Source: CAD feature listing. Evaluate the final solid. Frame: model axes, mm. A direction names the side the tool comes from. Round coordinates to 2 decimals unless told otherwise and drop trailing zeros. Write each loop counter-clockwise with the first axis right and the second up, starting at its lowest first coordinate (ties: lowest second). Pieces come first, ordered by that corner, then holes. Notation, with made-up numbers: (87.5, 49) -> (114.5, 49) arc R10 cw to (114.5, 64) -> close; hole circle Ø11 at (41.25, -0.75). An arc over 180 degrees is marked (long way). Put each result on its own line as item: value.
```python
from build123d import *

# Parameters (mm, degrees)
ESQUISSE1_W               = 60.5
ESQUISSE1_H               = 64
BOSS_EXTRU_1_DEPTH        = 30
ESQUISSE2_R               = 4.5
ENL_V_MAT_EXTRU_1_DEPTH   = 32
ENL_V_MAT_EXTRU_2_REACH   = 55.283
ESQUISSE4_W               = 52.1
ESQUISSE4_H               = 83.557669167
ESQUISSE5_R               = 10.5
ENL_V_MAT_EXTRU_3_DEPTH   = 1.7
ESQUISSE6_R               = 10
ENL_V_MAT_EXTRU_4_DEPTH   = 4.2
ESQUISSE7_W               = 47
ESQUISSE7_H               = 57
BOSS_EXTRU_2_DEPTH        = 30
ENL_V_MAT_EXTRU_5_DEPTH   = 30
ENL_V_MAT_EXTRU_6_DEPTH   = 8.25
ESQUISSE11_W              = 5
ESQUISSE11_H              = 40.5
BOSS_EXTRU_3_DEPTH        = 5
ESQUISSE12_R              = 0.5
ENL_V_MAT_EXTRU_7_DEPTH   = 15
TROU_TARAUD_M2X0_42_D     = 1.6
TROU_TARAUD_M2X0_42_DEPTH = 17
TROU_TARAUD_M2X0_42_TIP   = 0.480688495
ENL_V_MAT_EXTRU_8_REACH   = 113.72
TROU_TARAUD_M3X0_54_D     = 2.5
TROU_TARAUD_M3X0_54_DEPTH = 17.5
TROU_TARAUD_M3X0_54_TIP   = 0.751075774
ENL_V_MAT_EXTRU_9_REACH   = 100.671
ESQUISSE26_W              = 5
ESQUISSE26_H              = 64.513244551
BOSS_EXTRU_5_START        = 0.8
BOSS_EXTRU_5_DEPTH        = 0.8
BOSS_EXTRU_6_DEPTH        = 0.5
ESQUISSE30_R              = 10
ENL_V_MAT_EXTRU_10_DEPTH  = 20.5
ENL_V_START               = -20.5
ESQUISSE32_R              = 10.5
ENL_V_MAT_EXTRU_13_DEPTH  = 20.5


with BuildPart() as part:
    # Esquisse1 → Boss.-Extru.1 (new body)
    with BuildSketch(Plane.XY):
        Rectangle(ESQUISSE1_W, ESQUISSE1_H)
    extrude(amount=BOSS_EXTRU_1_DEPTH)

    # Esquisse2 → Enlèv. mat.-Extru.1 (cut)
    with BuildSketch(Plane(origin=(30.25, 0, 0), x_dir=(0, 0, -1), z_dir=(1, 0, 0))):
        with Locations(Location((-15, -17, 0), (0, 0, 90))):
            Circle(ESQUISSE2_R)
    extrude(amount=-ENL_V_MAT_EXTRU_1_DEPTH, mode=Mode.SUBTRACT)

    # Enlèv. mat.-Extru.2: up to this face of the body (flat: up to its plane)
    enl_v_mat_extru_2_end = Plane(part.part.faces().sort_by_distance((0, 0, 0))[0])
    # Esquisse4 → Enlèv. mat.-Extru.2 (cut, up to the picked face)
    with BuildSketch(Plane.XY.offset(30), mode=Mode.PRIVATE) as enl_v_mat_extru_2_sk1:
        with Locations((0, -14.778834584)):
            Rectangle(ESQUISSE4_W, ESQUISSE4_H)
    enl_v_mat_extru_2_tool1 = split(extrude(enl_v_mat_extru_2_sk1.sketch, amount=-ENL_V_MAT_EXTRU_2_REACH, mode=Mode.PRIVATE), bisect_by=enl_v_mat_extru_2_end, keep=Keep.BOTH, mode=Mode.PRIVATE)
    add(enl_v_mat_extru_2_tool1.solids().sort_by(Axis((0, -14.778835, 30), (0, 0, -1)))[0], mode=Mode.SUBTRACT)

    # Esquisse5 → Enlèv. mat.-Extru.3 (cut)
    with BuildSketch(Plane(origin=(30.25, 0, 0), x_dir=(0, 0, -1), z_dir=(1, 0, 0))):
        with Locations(Location((-15, -17, 0), (0, 0, 90))):
            Circle(ESQUISSE5_R)
    extrude(amount=-ENL_V_MAT_EXTRU_3_DEPTH, mode=Mode.SUBTRACT)

    # Esquisse6 → Enlèv. mat.-Extru.4 (cut)
    with BuildSketch(Plane(origin=(-26.05, 0, 0), x_dir=(0, 0, -1), z_dir=(1, 0, 0))):
        with Locations((-15, -17)):
            Circle(ESQUISSE6_R)
    extrude(amount=-ENL_V_MAT_EXTRU_4_DEPTH, mode=Mode.SUBTRACT)

    # Esquisse7 → Boss.-Extru.2 (add)
    with BuildSketch(Plane.XY.offset(30)):
        with Locations((-6.75, 60.5)):
            Rectangle(ESQUISSE7_W, ESQUISSE7_H)
    extrude(amount=-BOSS_EXTRU_2_DEPTH)

    # Esquisse8 → Enlèv. mat.-Extru.5 (cut)
    with BuildSketch(Plane.XY.offset(30)):
        Polygon((-15.25, 80.75), (11.75, 80.75), (11.75, 98.556441221), (21.75, 98.556441221), (21.75, 32), (11.75, 32), (11.75, 40.25), (-15.25, 40.25), align=None)
    extrude(amount=-ENL_V_MAT_EXTRU_5_DEPTH, mode=Mode.SUBTRACT)

    # Esquisse10 → Enlèv. mat.-Extru.6 (cut)
    with BuildSketch(Plane.XZ.offset(-80.75)):
        Polygon((-5.25, 11), (-5.25, 12), (34.75, 12), (34.75, 18), (-5.25, 18), (-5.25, 19), (-15.25, 19), (-15.25, 11), align=None)
    extrude(amount=-ENL_V_MAT_EXTRU_6_DEPTH, mode=Mode.SUBTRACT)

    # Esquisse11 → Boss.-Extru.3 (add)
    with BuildSketch(Plane(origin=(-15.25, 0, 0), x_dir=(0, 0, -1), z_dir=(1, 0, 0))):
        with Locations((-27.5, 60.5)):
            Rectangle(ESQUISSE11_W, ESQUISSE11_H)
        with Locations((-2.5, 60.5)):
            Rectangle(ESQUISSE11_W, ESQUISSE11_H)
    extrude(amount=BOSS_EXTRU_3_DEPTH)

    # Esquisse12 → Enlèv. mat.-Extru.7 (cut)
    with BuildSketch(Plane(origin=(11.75, 0, 0), x_dir=(0, 0, -1), z_dir=(1, 0, 0))):
        with Locations((-19.925, 85.21)):
            Circle(ESQUISSE12_R)
        with Locations(Location((-10.075, 85.21, 0), (0, 0, 180))):
            Circle(ESQUISSE12_R)
        with Locations((-10.075, 35.79)):
            Circle(ESQUISSE12_R)
        with Locations(Location((-19.925, 35.79, 0), (0, 0, 180))):
            Circle(ESQUISSE12_R)
    extrude(amount=-ENL_V_MAT_EXTRU_7_DEPTH, mode=Mode.SUBTRACT)

    # Trou taraudé M2x0.42
    with Locations(Plane(origin=(11.75, 85.21, 19.925), x_dir=(0, 0, 1), z_dir=(1, 0, 0))):
        with Locations((0, 0), (-9.85, 0), (-9.85, 49.42), (0, 49.42)):
            Hole(TROU_TARAUD_M2X0_42_D / 2, depth=TROU_TARAUD_M2X0_42_DEPTH)
            with Locations((0, 0, -(TROU_TARAUD_M2X0_42_DEPTH + TROU_TARAUD_M2X0_42_TIP / 2))):  # 118° drill point
                Cone(0, TROU_TARAUD_M2X0_42_D / 2, TROU_TARAUD_M2X0_42_TIP, mode=Mode.SUBTRACT)

    # Enlèv. mat.-Extru.8: up to this face of the body (flat: up to its plane)
    enl_v_mat_extru_8_end = Plane(part.part.faces().sort_by_distance((30.25, 3.741727612, 15))[0])
    # Esquisse15 → Enlèv. mat.-Extru.8 (cut, up to the picked face)
    with BuildSketch(Plane.ZY.offset(30.25), mode=Mode.PRIVATE) as enl_v_mat_extru_8_sk1:
        with BuildLine():
            Line((40, -17), (30, -17))
            ThreePointArc((30, -17), (15, -32), (0, -17))
            Line((0, -17), (-10, -17))
            ThreePointArc((-10, -17), (15, -42), (40, -17))
        make_face()
    enl_v_mat_extru_8_tool1 = split(extrude(enl_v_mat_extru_8_sk1.sketch, amount=-ENL_V_MAT_EXTRU_8_REACH, mode=Mode.PRIVATE), bisect_by=enl_v_mat_extru_8_end, keep=Keep.BOTH, mode=Mode.PRIVATE)
    add(enl_v_mat_extru_8_tool1.solids().sort_by(Axis((-30.25, -17.559017, -5), (1, 0, 0)))[0], mode=Mode.SUBTRACT)

    # Trou taraudé M3x0.54
    with Locations(Plane(origin=(-30.25, 70.15, 15), x_dir=(0, -1, 0), z_dir=(-1, 0, 0))):
        with Locations((0, 0)):
            Hole(TROU_TARAUD_M3X0_54_D / 2, depth=TROU_TARAUD_M3X0_54_DEPTH)
            with Locations((0, 0, -(TROU_TARAUD_M3X0_54_DEPTH + TROU_TARAUD_M3X0_54_TIP / 2))):  # 118° drill point
                Cone(0, TROU_TARAUD_M3X0_54_D / 2, TROU_TARAUD_M3X0_54_TIP, mode=Mode.SUBTRACT)

    # Enlèv. mat.-Extru.9: up to this face of the body (flat: up to its plane)
    enl_v_mat_extru_9_end = Plane(part.part.faces().sort_by_distance((-10.488138476, 46.757965151, 0))[0])
    # Esquisse26 → Enlèv. mat.-Extru.9 (cut, up to the picked face)
    with BuildSketch(Plane.XY.offset(30), mode=Mode.PRIVATE) as enl_v_mat_extru_9_sk1:
        with Locations((-27.75, 64.256622276)):
            Rectangle(ESQUISSE26_W, ESQUISSE26_H)
    enl_v_mat_extru_9_tool1 = split(extrude(enl_v_mat_extru_9_sk1.sketch, amount=-ENL_V_MAT_EXTRU_9_REACH, mode=Mode.PRIVATE), bisect_by=enl_v_mat_extru_9_end, keep=Keep.BOTH, mode=Mode.PRIVATE)
    add(enl_v_mat_extru_9_tool1.solids().sort_by(Axis((-27.75, 64.256622, 30), (0, 0, -1)))[0], mode=Mode.SUBTRACT)

    # Esquisse27 → Boss.-Extru.5 (add)
    with BuildSketch(Plane.ZY.offset(30.25).offset(BOSS_EXTRU_5_START)):
        with BuildLine():
            Line((30, -17), (30, 32))
            Line((30, 32), (0, 32))
            Line((0, 32), (0, -17))
            ThreePointArc((0, -17), (15, -32), (30, -17))
        make_face()
    extrude(amount=-BOSS_EXTRU_5_DEPTH)

    # Esquisse28 → Boss.-Extru.6 (add)
    with BuildSketch(Plane(origin=(30.25, 0, 0), x_dir=(0, 0, -1), z_dir=(1, 0, 0))):
        with BuildLine():
            Line((-30, 32), (-30, -17))
            ThreePointArc((-30, -17), (-15, -32), (0, -17))
            Line((0, -17), (0, 32))
            Line((0, 32), (-30, 32))
        make_face()
    extrude(amount=BOSS_EXTRU_6_DEPTH)

    # Esquisse30 → Enlèv. mat.-Extru.10 (cut)
    with BuildSketch(Plane(origin=(-30.25, 0, 0), x_dir=(0, 0, -1), z_dir=(1, 0, 0))):
        with Locations((-15, -17)):
            Circle(ESQUISSE30_R)
    extrude(amount=-ENL_V_MAT_EXTRU_10_DEPTH, mode=Mode.SUBTRACT)

    # Esquisse32 → Enlèv. mat.-Extru.13 (cut)
    with BuildSketch(Plane.ZY.offset(-30.25).offset(ENL_V_START)):
        with Locations(Location((15, -17, 0), (0, 0, 90))):
            Circle(ESQUISSE32_R)
    extrude(amount=ENL_V_MAT_EXTRU_13_DEPTH, mode=Mode.SUBTRACT)


solid = part.part
```
Q1. Cut plane B-B on y = 1.5. Output: boundary loops of the cut face in (x, z).
Ans:
outline: (-31.05, 0) -> (-26.05, 0) -> (-26.05, 30) -> (-31.05, 30) -> close; (26.05, 0) -> (30.75, 0) -> (30.75, 30) -> (26.05, 30) -> close
Q2. Material intervals for line 1 (Z direction, x = 8, y = 85.21) (3 decimals); line 2 (Z direction, x = 7, y = 35.79) (3 decimals); line 3 (Z direction, x = 1, y = 85), sorted ascending. Write a range as [from, to].
Ans:
line 1: z = [0, 9.275], [10.875, 12], [18, 19.125], [20.725, 30]
line 2: z = [0, 9.275], [10.875, 19.125], [20.725, 30]
line 3: z = [0, 9.3], [10.85, 12], [18, 19.15], [20.7, 30]
Q3. Pin query (flat end, axial travel): pin 1 (1.3 mm diameter, centred on y = 35.79, z = 19.925, fed in from -X); pin 2 (9 mm diameter, centred on y = 83.5, z = 24.5, fed in from +X); pin 3 (3 mm diameter, centred on x = 1.5, z = 12, fed in from -Y). Return the tip coordinate at first contact, or that it passes through.
Ans:
pin 1: stops at x = -25.25
pin 2: stops at x = 11.75
pin 3: stops at y = 27
Q4. Reachability of faces 4 (the flat face through (-10.25, 61, 28)), 5 (the cylindrical face through (29.665, -12.155, 24.315)), 6 (the flat face through (3, 85, 18)), 7 (the flat face through (21, 32, 15)) from +Z, -Z, +X, -X, +Y, -Y: full face, straight path, thin tool, end or side. Return the list, or none.
Ans:
face 4: +Z, -Z, +X
face 5: +X
face 6: +X, +Y
face 7: +Z, -Z, +X, +Y
Q5. Draft query along Y for faces 1 (the flat face through (-2, 40.25, 15)), 2 (the flat face through (-3, 89, 19)), 3 (the flat face through (-10, 85, 19)). Return one class per face: +Y half, -Y half, draft (parallel to the pull), parting line (faces both ways), or undercut.
Ans:
face 1: undercut
face 2: +Y half
face 3: draft
Q6. Cut plane A-A on x = -1. Output: boundary loops of the cut face in (y, z) (3 decimals).
Ans:
outline: (27, 0) -> (40.25, 0) -> (40.25, 30) -> (27, 30) -> close; (80.75, 0) -> (89, 0) -> (89, 12) -> (80.75, 12) -> close; (80.75, 18) -> (89, 18) -> (89, 30) -> (80.75, 30) -> close; hole circle Ø1.6 at (35.79, 10.075); hole circle Ø1.6 at (35.79, 19.925); hole circle Ø1.6 at (85.21, 10.075); hole circle Ø1.6 at (85.21, 19.925)
Q7. Cut plane C-C on z = 15. Give the number of separate pieces and of enclosed holes in the cut face, and give its area (3 significant figures).
Ans:
separate pieces: 4
enclosed holes: 0
area: 1,480 mm^2
Q8. Cut plane D-D on z = 6.75. Output: boundary loops of the cut face in (x, y), and give its area (3 significant figures).
Ans:
outline: (-31.05, -29.53) -> (-26.05, -29.53) -> (-26.05, -22.65) -> (-31.05, -22.65) -> close; (-31.05, -11.35) -> (-26.05, -11.35) -> (-26.05, 27) -> (26.05, 27) -> (26.05, -29.53) -> (30.75, -29.53) -> (30.75, -23.5) -> (28.55, -23.5) -> (28.55, -10.5) -> (30.75, -10.5) -> (30.75, 32) -> (11.75, 32) -> (11.75, 40.25) -> (-15.25, 40.25) -> (-15.25, 80.75) -> (11.75, 80.75) -> (11.75, 89) -> (-25.25, 89) -> (-25.25, 32) -> (-31.05, 32) -> close
area: 1,790 mm^2
